from build123d import *

# Parameters (mm, degrees)
F1_DEPTH = 7.62
F3_DEPTH = 5.08
F4_W     = 10.16
F4_H     = 1.748005039
F5_DEPTH = 5.08


# Not quite as in the source:
# - a feature names something its author has since deleted; it is built from what else it names


with BuildPart() as f1:
    # F0 (on Top) → F1 (new body)
    with BuildSketch(Plane.XY):
        Polygon((-11.43, -15.732045351), (11.43, -15.732045351), (18.4941284914, 6.0091066115), (0, 19.4458774789), (-18.4941284914, 6.0091066115), align=None)
    extrude(amount=F1_DEPTH)

    # F2 (on Top) → F3 (cut)
    with BuildSketch(Plane.XY):
        Polygon((10.16, -13.984040312), (16.4392253257, 5.3414280991), (0, 17.2852244257), (-16.4392253257, 5.3414280991), (-10.16, -13.984040312), align=None)
    extrude(amount=F3_DEPTH, mode=Mode.SUBTRACT)

    # F4 (on face) → F5 (cut)
    with BuildSketch(Plane(origin=(0, 0, 0), x_dir=(1, 0, 0), z_dir=(0, 0, -1))):
        Polygon((-14.8694189943, -0.5100609964), (-13.2996126628, 4.3213061064), (-14.9620642457, 4.8614693697), (-16.5318705771, 0.030102267), align=None)
        Polygon((-14.9620642457, 4.8614693697), (-13.2996126628, 4.3213061064), (-11.7298063314, 9.1526732092), (-13.3922579143, 9.6928364725), align=None)
        Polygon((11.7298063314, 9.1526732092), (13.2996126628, 4.3213061064), (14.9620642457, 4.8614693697), (13.3922579143, 9.6928364725), align=None)
        Polygon((14.9620642457, 4.8614693697), (13.2996126628, 4.3213061064), (14.8694189943, -0.5100609964), (16.5318705771, 0.030102267), align=None)
        with Locations((0, 14.8580428315)):
            Rectangle(F4_W, F4_H)
        Polygon((0, -19.4458774789), (0, -17.2852244257), (-11.3019674114, -9.0738644512), (-12.3294189943, -10.488030234), align=None)
        Polygon((11.3019674114, -9.0738644512), (0, -17.2852244257), (0, -19.4458774789), (12.3294189943, -10.488030234), align=None)
    extrude(amount=-F5_DEPTH, mode=Mode.SUBTRACT)


solid = f1.part
Can you work these out from the model? Positions are in its coordinate system, mm. A direction names the side the tool comes from. Round coordinates to 2 decimals unless told otherwise and drop trailing zeros. Write each loop counter-clockwise with the first axis right and the second up, starting at its lowest first coordinate (ties: lowest second). Pieces come first, ordered by that corner, then holes. Notation, with made-up numbers: M 55.5,-29.5 L 72.5,-29.5 A25 cw 72.5,0.5 Z; hole C -35,89 d2. An arc over 180 degrees is marked long. Use a Markdown table: item, result.
Item 1: We'd pull the mould along Y, two halves only. Please class faces 4 (the face through (11.82, 9.79, 2.5)), 5 (the face through (14.913, -5.014, 5.45)), 6 (the face through (-15.665, 2.96, 2.504)): released by +Y, released by -Y, zero draft, split by the parting line, or undercut.
Found:
| item | result |
|---|---|
| face 4 | released by +Y |
| face 5 | released by -Y |
| face 6 | undercut |
Item 2: I want a section at D-D (x = 9). List the corners of the cut face in (y, z) for me.
Found:
| item | result |
|---|---|
| outline | M -15.73,0 L -13.98,0 L -13.98,5.08 L 12.91,5.08 L 12.91,7.62 L -15.73,7.62 Z |
Item 3: For pin 1 Ø10 at (x, y) = (-6.5, -1.5) entering from -Z; pin 2 Ø2.5 at (x, z) = (7, 3) entering from +Y; pin 3 Ø1.5 at (y, z) = (4, 6) entering from +X (3 decimals); pin 4 Ø1 at (y, z) = (15.5, 3.5) entering from -X, each with a flat end and sliding along its axis, tell me the tip position at first contact or that it passes through.
Found:
| item | result |
|---|---|
| pin 1 | stops at z = 5.08 |
| pin 2 | stops at y = -13.98 |
| pin 3 | stops at x = 18.085 |
| pin 4 | passes through |
Item 4: I want a section at B-B (y = -13). List the corners of the cut face in (x, z) for me.
Found:
| item | result |
|---|---|
| outline | M -12.32,0 L -10.48,0 L -10.48,5.08 L 10.48,5.08 L 10.48,0 L 12.32,0 L 12.32,7.62 L -12.32,7.62 Z |
Item 5: I want a section at C-C (z = 6). List the corners of the cut face in (x, y) for me, and give its area (3 significant figures).
Found:
| item | result |
|---|---|
| outline | M -18.49,6.01 L -11.43,-15.73 L 11.43,-15.73 L 18.49,6.01 L 0,19.45 Z |
| area | 899 mm2 |
Item 6: I want a section at A-A (z = 4). List the corners of the cut face in (x, y) for me, and give its area (3 significant figures).
Found:
| item | result |
|---|---|
| outline | M -18.49,6.01 L -16.53,-0.03 L -14.87,0.51 L -16.44,5.34 L -11.3,9.07 L -12.33,10.49 Z; M -13.39,-9.69 L -11.43,-15.73 L -5.08,-15.73 L -5.08,-13.98 L -10.16,-13.98 L -11.73,-9.15 Z; M 5.08,-15.73 L 11.43,-15.73 L 13.39,-9.69 L 11.73,-9.15 L 10.16,-13.98 L 5.08,-13.98 Z; M 11.3,9.07 L 16.44,5.34 L 14.87,0.51 L 16.53,-0.03 L 18.49,6.01 L 12.33,10.49 Z |
| area | 84.4 mm2 |
Item 7: Which directions (+Z, -Z, +X, -X, +Y, -Y) give clear straight access to the entire face, cutting with the end or side of a thin tool? Please do faces 1 (the face through (5.08, -15, 3)), 2 (the face through (-12.55, -9.42, 2.5)), 3 (the face through (-8, -13.984, 3)).
Found:
| item | result |
|---|---|
| face 1 | -Z, +Y, -Y |
| face 2 | -Z, -X |
| face 3 | -Z, +Y |
Item 8: If I drill on line 1 along Z through (x, y) = (-4, 3.5); line 2 along X through (y, z) = (9, 1.5); line 3 along Y through (x, z) = (-8.5, 4), over which ranges is the centre line in solid material (lowest first)? Write a range as [from, to].
Found:
| item | result |
|---|---|
| line 1 | z = [5.08, 7.62] |
| line 2 | x = [-14.38, -11.4], [11.4, 14.38] |
| line 3 | y = [-15.73, -13.98] |
